For this review, use the dimensioned drawing (mm, ordinates from the lowest corner) and the shaded views. Give positions to 0.01 mm unless a question says otherwise; leave off trailing zeros. Order: outer loops, then holes, each group sorted by start corner. A loop starts at its lowest first (then second) coordinate and runs counter-clockwise, first axis right, second up.
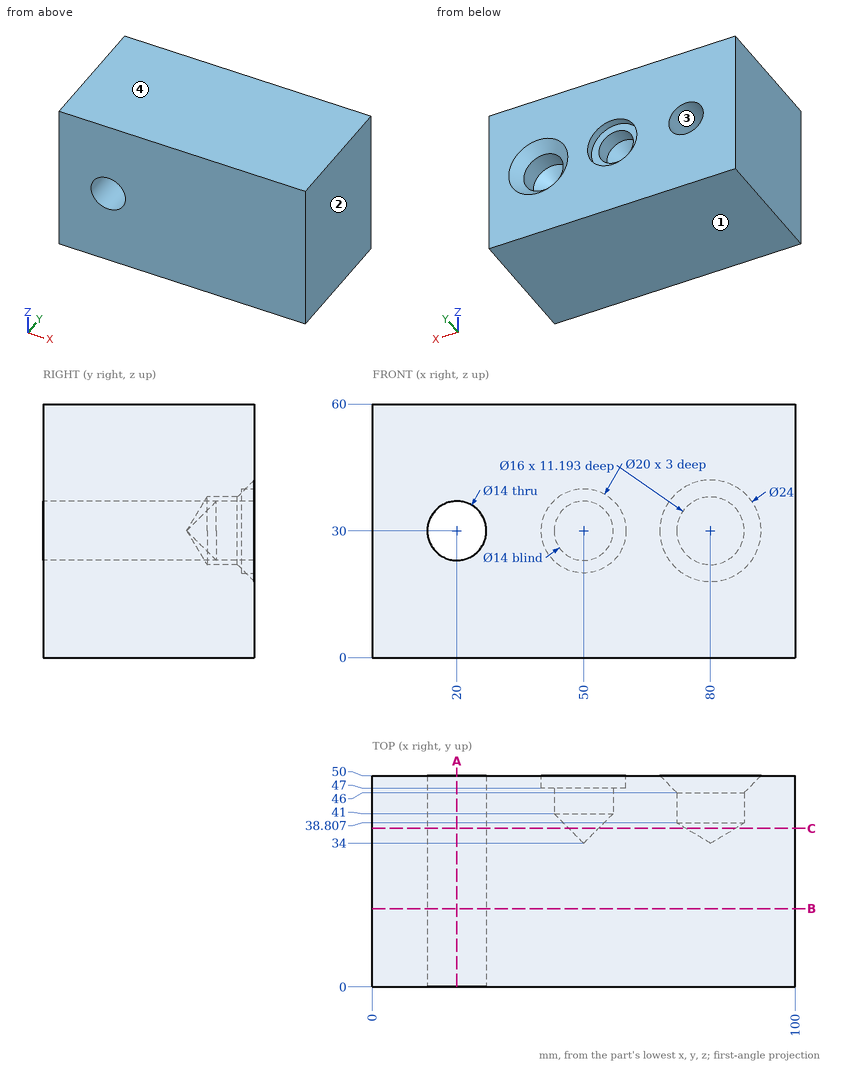
1. Take a section at C-C (y = 37.5). Write out the cut boundary in (x, z) (3 decimals), and give its area (3 significant figures).
2. Draft analysis for pull direction Z (two halves, no side actions). For the marked faces 1, 2, 3 and 4, state which applies: pulls with the +Z half, pulls with the -Z half, needs draft (parallel to the pull), parting line crosses it, or undercut.
3. Take a section at B-B (y = 18.5). Write out the cut boundary in (x, z).
4. To check wall thickness, follow line 1 (X direction, y = 16.5, z = 30); line 2 (Z direction, x = 50, y = 44); line 3 (Z direction, x = 50, y = 47.65). State the ranges of each line that lie inside material, in increasing order.
5. Insertion check: pin 1 (18.5 mm diameter, centred on x = 80, z = 30, fed in from +Y); pin 2 (1 mm diameter, centred on x = 46.5, z = 38, fed in from +Y); pin 3 (8.5 mm diameter, centred on x = 20, z = 30, fed in from -Y). Each pin has a flat end and moves straight along its axis. Give the tip position at first contact, or say it passes through.
6. Take a section at A-A (x = 20). Write out the cut boundary in (y, z), and give its area (3 significant figures).
Answer:
1. outline: (0, 0) - (100, 0) - (100, 60) - (0, 60) - close; hole circle Ø14 at (20, 30); hole circle Ø7 at (50, 30); hole circle Ø11.65 at (80, 30)
1. area: 5,700 mm2
2. face 1: pulls with the -Z half
2. face 2: needs draft
2. face 3: undercut
2. face 4: pulls with the +Z half
3. outline: (0, 0) - (100, 0) - (100, 60) - (0, 60) - close; hole circle Ø14 at (20, 30)
4. line 1: x = 0 to 13, 27 to 100
4. line 2: z = 0 to 23, 37 to 60
4. line 3: z = 0 to 20, 40 to 60
5. pin 1: stops at y = 47.25
5. pin 2: stops at y = 47
5. pin 3: passes through
6. outline: (0, 0) - (50, 0) - (50, 23) - (0, 23) - close; (0, 37) - (50, 37) - (50, 60) - (0, 60) - close
6. area: 2,300 mm2
